Verification items for the finished model (mm, model axes). Face numbers are marked on the shaded views. A direction names the side the tool comes from. Round coordinates to 2 decimals unless told otherwise and drop trailing zeros. Loops run counter-clockwise (first coordinate to the right, second up) from the corner with the lowest first, then second, coordinate; pieces in that order, holes last.
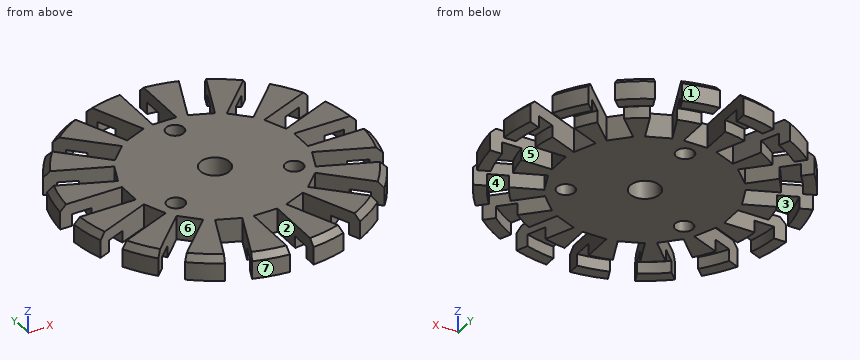
from build123d import *

# Parameters (mm, degrees)
ESBO_O1_R             = 25
EXTRUS_O1_DEPTH       = 4
EXTRUS_O2_DEPTH       = 1
EXTRUS_O2_DEPTH_BACK  = 5
CHANFRO1_SIZE         = 1
CIRPATTERN1_COUNT     = 16
ESBO_O5_R             = 1.5
ESBO_O5_R_2           = 2.5
CORTE_EXTRUS_O2_DEPTH = 36.468295702
ESBO_O8_R             = 23
ESBO_O8_R_2           = 19.75
CORTE_EXTRUS_O4_DEPTH = 2


with BuildPart() as part:
    # Esbo_o1 → Extrus_o1 (new body)
    with BuildSketch(Plane.XY):
        Circle(ESBO_O1_R)
    extrude(amount=EXTRUS_O1_DEPTH)

    # Chanfro1
    chanfro1_edges = [part.edges().sort_by_distance(p)[0] for p in [
        (-25, 0, 4),
    ]]
    chamfer(chanfro1_edges, length=CHANFRO1_SIZE)


with BuildPart() as body_2:
    # Esbo_o2 → Extrus_o2 (new, two sides: drawn at the far end of the back side and taken through both)
    with BuildSketch(Plane.XY.offset(4).offset(-EXTRUS_O2_DEPTH_BACK)):
        Polygon((0, 14.5), (2, 14.5), (2, 29.5), (-2, 29.5), (-2, 14.5), align=None)
    extrude(amount=EXTRUS_O2_DEPTH + EXTRUS_O2_DEPTH_BACK)


with BuildPart() as cirpattern1_1:
    # CirPattern1: pattern copy
    add(body_2.part.rotate(Axis((0, 0, 0), (0, 0, 1)), 1 * 360 / CIRPATTERN1_COUNT))


with BuildPart() as cirpattern1_2:
    # CirPattern1: pattern copy
    add(body_2.part.rotate(Axis((0, 0, 0), (0, 0, 1)), 2 * 360 / CIRPATTERN1_COUNT))


with BuildPart() as cirpattern1_3:
    # CirPattern1: pattern copy
    add(body_2.part.rotate(Axis((0, 0, 0), (0, 0, 1)), 3 * 360 / CIRPATTERN1_COUNT))


with BuildPart() as cirpattern1_4:
    # CirPattern1: pattern copy
    add(body_2.part.rotate(Axis((0, 0, 0), (0, 0, 1)), 4 * 360 / CIRPATTERN1_COUNT))


with BuildPart() as cirpattern1_5:
    # CirPattern1: pattern copy
    add(body_2.part.rotate(Axis((0, 0, 0), (0, 0, 1)), 5 * 360 / CIRPATTERN1_COUNT))


with BuildPart() as cirpattern1_6:
    # CirPattern1: pattern copy
    add(body_2.part.rotate(Axis((0, 0, 0), (0, 0, 1)), 6 * 360 / CIRPATTERN1_COUNT))


with BuildPart() as cirpattern1_7:
    # CirPattern1: pattern copy
    add(body_2.part.rotate(Axis((0, 0, 0), (0, 0, 1)), 7 * 360 / CIRPATTERN1_COUNT))


with BuildPart() as cirpattern1_8:
    # CirPattern1: pattern copy
    add(body_2.part.rotate(Axis((0, 0, 0), (0, 0, 1)), 8 * 360 / CIRPATTERN1_COUNT))


with BuildPart() as cirpattern1_9:
    # CirPattern1: pattern copy
    add(body_2.part.rotate(Axis((0, 0, 0), (0, 0, 1)), 9 * 360 / CIRPATTERN1_COUNT))


with BuildPart() as cirpattern1_10:
    # CirPattern1: pattern copy
    add(body_2.part.rotate(Axis((0, 0, 0), (0, 0, 1)), 10 * 360 / CIRPATTERN1_COUNT))


with BuildPart() as cirpattern1_11:
    # CirPattern1: pattern copy
    add(body_2.part.rotate(Axis((0, 0, 0), (0, 0, 1)), 11 * 360 / CIRPATTERN1_COUNT))


with BuildPart() as cirpattern1_12:
    # CirPattern1: pattern copy
    add(body_2.part.rotate(Axis((0, 0, 0), (0, 0, 1)), 12 * 360 / CIRPATTERN1_COUNT))


with BuildPart() as cirpattern1_13:
    # CirPattern1: pattern copy
    add(body_2.part.rotate(Axis((0, 0, 0), (0, 0, 1)), 13 * 360 / CIRPATTERN1_COUNT))


with BuildPart() as cirpattern1_14:
    # CirPattern1: pattern copy
    add(body_2.part.rotate(Axis((0, 0, 0), (0, 0, 1)), 14 * 360 / CIRPATTERN1_COUNT))


with BuildPart() as cirpattern1_15:
    # CirPattern1: pattern copy
    add(body_2.part.rotate(Axis((0, 0, 0), (0, 0, 1)), 15 * 360 / CIRPATTERN1_COUNT))


with BuildPart() as part_1:
    add(part.part)

    # Combinar1: cut CirPattern1_1, body 2, CirPattern1_15, CirPattern1_14, CirPattern1_13, CirPattern1_12, CirPattern1_11, CirPattern1_10, CirPattern1_9, CirPattern1_8, CirPattern1_7, CirPattern1_6, CirPattern1_5, CirPattern1_4, CirPattern1_3, CirPattern1_2
    add(cirpattern1_1.part, mode=Mode.SUBTRACT)
    add(body_2.part, mode=Mode.SUBTRACT)
    add(cirpattern1_15.part, mode=Mode.SUBTRACT)
    add(cirpattern1_14.part, mode=Mode.SUBTRACT)
    add(cirpattern1_13.part, mode=Mode.SUBTRACT)
    add(cirpattern1_12.part, mode=Mode.SUBTRACT)
    add(cirpattern1_11.part, mode=Mode.SUBTRACT)
    add(cirpattern1_10.part, mode=Mode.SUBTRACT)
    add(cirpattern1_9.part, mode=Mode.SUBTRACT)
    add(cirpattern1_8.part, mode=Mode.SUBTRACT)
    add(cirpattern1_7.part, mode=Mode.SUBTRACT)
    add(cirpattern1_6.part, mode=Mode.SUBTRACT)
    add(cirpattern1_5.part, mode=Mode.SUBTRACT)
    add(cirpattern1_4.part, mode=Mode.SUBTRACT)
    add(cirpattern1_3.part, mode=Mode.SUBTRACT)
    add(cirpattern1_2.part, mode=Mode.SUBTRACT)

    # Esbo_o5 → Corte-extrus_o2 (cut, through all)
    with BuildSketch(Plane.XY.offset(4)):
        with Locations((0, 11.5)):
            Circle(ESBO_O5_R)
        with Locations((9.959292144, -5.75)):
            Circle(ESBO_O5_R)
        with Locations((-9.959292144, -5.75)):
            Circle(ESBO_O5_R)
        Circle(ESBO_O5_R_2)
    extrude(amount=-CORTE_EXTRUS_O2_DEPTH, mode=Mode.SUBTRACT)

    # Esbo_o8 → Corte-extrus_o4 (cut)
    with BuildSketch(Plane(origin=(0, 0, 0), x_dir=(-1, 0, 0), z_dir=(0, 0, -1))):
        Circle(ESBO_O8_R)
        Circle(ESBO_O8_R_2, mode=Mode.SUBTRACT)
    extrude(amount=-CORTE_EXTRUS_O4_DEPTH, mode=Mode.SUBTRACT)


solid = part_1.part
1. Scan lines: L1, parallel to Y at x = 0, z = 2.25; L2, parallel to X at y = 17.5, z = 2.3; L3, parallel to Y at x = 14, z = 3.7. Record each from-to range of solid material in increasing order.
2. Tool access check on the marked faces 4, 5, 6 and 7. Record the directions out of +Z, -Z, +X, -X, +Y, -Y that give a thin tool (end or side, any length) a straight path to the whole face; none if there is none.
3. Section check B-B (y = 0). Enter the section's corners in (x, z).
4. Section check C-C (z = 0.85). Give the number of separate pieces and of enclosed holes in the cut face, then the cut area to 3 significant figures.
5. Gauge pin test, flat ends, axial feed: P1, Ø2.5, axis at x = -12.5, y = 17, coming from the -Z side; P2, Ø1.2, axis at y = -1, z = 3, coming from the -X side; P3, Ø1.5, axis at x = -13.5, y = 1, coming from the -Z side; P4, Ø2, axis at x = -21.5, z = 2.5, coming from the -Y side. Record the tip position at first contact, or that the pin passes through.
6. Section check A-A (x = 0). Enter the section's corners in (y, z).
7. Release check for a two-part mould opening along Y. For the marked faces 1, 2 and 3 record: released by +Y, released by -Y, zero draft, split by the parting line, or undercut.
Taken from the geometry:
1. L1: y = -14.5 to -2.5, 2.5 to 10, 13 to 14.5
1. L2: x = -14.67 to -9.41, -5.08 to -2, 2 to 5.08, 9.41 to 14.67
1. L3: y = -19.86 to -16.83, -11.17 to -7.96, -4.09 to 4.09, 7.96 to 11.17, 16.83 to 19.86
2. face 4: -Z
2. face 5: +Z, -Z, +X
2. face 6: +Z, -Z
2. face 7: +Z, -Z, -X, -Y
3. outline: (-14.5, 0) - (-2.5, 0) - (-2.5, 4) - (-14.5, 4) - close; (2.5, 0) - (14.5, 0) - (14.5, 4) - (2.5, 4) - close
4. separate pieces: 17
4. enclosed holes: 4
4. area: 1,020 mm2
5. P1: stops at z = 2
5. P2: stops at x = -14.5
5. P3: stops at z = 0
5. P4: stops at y = -14.31
6. outline: (-14.5, 0) - (-2.5, 0) - (-2.5, 4) - (-14.5, 4) - close; (2.5, 0) - (10, 0) - (10, 4) - (2.5, 4) - close; (13, 0) - (14.5, 0) - (14.5, 4) - (13, 4) - close
7. face 1: released by +Y
7. face 2: zero draft
7. face 3: undercut
